Geometry: final body of the model. Coordinates: model frame, mm. Coordinates: 2 decimals unless noted, no trailing zeros. Write each loop counter-clockwise with the first axis right and the second up, starting at its lowest first coordinate (ties: lowest second). Pieces come first, ordered by that corner, then holes. Notation, with made-up numbers: (-15.75, 81) - (7.25, 81) arc R23 cw to (7.25, 104) - close; hole circle Ø5 at (70.5, 45.5). An arc over 180 degrees is marked (long way). Answer as a JSON object with one key per item and string values. Group by question number.
Item 1: Section B-B on x = -9. Return loops of the section in (y, z), and give its area (3 significant figures).
Item 2: First-contact query: pin 1 Ø2 at (x, y) = (18.5, -10.5) entering from -Z; pin 2 Ø6 at (x, y) = (12, -24) entering from +Z; pin 3 Ø8 at (x, y) = (32.5, -18.5) entering from -Z. Flat tips, straight axial feed; report the tip coordinate or a pass-through.
Item 3: Section C-C on z = -11. Return loops of the section in (x, y).
Item 4: Section A-A on y = -25.5. Return loops of the section in (x, z), and give its area (3 significant figures).
Item 5: Line query: line 1 along X through (y, z) = (-38.5, -6.5); line 2 along Z through (x, y) = (8, -37); line 3 along X through (y, z) = (-36.5, 7). Output: solid intervals per line, ascending. Write a range as from..to.
```python
from build123d import *

# Parameters (mm, degrees)
F1_DEPTH = 50.8


with BuildPart() as f1:
    # F0 (on Front) → F1 (new body)
    with BuildSketch(Plane.XZ):
        with BuildLine():
            Line((4.744167, 14.229999), (0, 15))
            ThreePointArc((0, 15), (-15, 0), (0, -15))
            Line((0, -15), (5.124627, -14.097454))
            ThreePointArc((5.124627, -14.097454), (12.285548, -8.60612), (15, 0))
            ThreePointArc((15, 0), (12.168864, 8.770333), (4.744167, 14.229999))
        make_face()
        with BuildLine():
            ThreePointArc((4.744167, 14.229999), (2.403124, 14.806248), (0, 15))
            Line((0, 15), (4.744167, 14.229999))
        make_face()
        with BuildLine():
            Line((5.124627, -14.097454), (0, -15))
            ThreePointArc((0, -15), (2.601749, -14.77264), (5.124627, -14.097454))
        make_face()
        with BuildLine():
            Line((31.602083, 9.870832), (4.744167, 14.229999))
            ThreePointArc((4.744167, 14.229999), (12.168864, 8.770333), (15, 0))
            ThreePointArc((15, 0), (12.285548, -8.60612), (5.124627, -14.097454))
            Line((5.124627, -14.097454), (28.800074, -9.927748))
            ThreePointArc((28.800074, -9.927748), (20.098668, 1.401293), (31.602083, 9.870832))
        make_face()
        with BuildLine():
            ThreePointArc((36.268126, 7.7917), (34.070104, 9.134235), (31.602083, 9.870832))
            ThreePointArc((31.602083, 9.870832), (20.098668, 1.401293), (28.800074, -9.927748))
            ThreePointArc((28.800074, -9.927748), (36.633277, -7.48329), (40, 0))
            ThreePointArc((40, 0), (39.018904, 4.319649), (36.268126, 7.7917))
        make_face()
    extrude(amount=F1_DEPTH)


solid = f1.part
```
Checks:
{
 "1": {"outline": "(-50.8, -12) - (0, -12) - (0, 12) - (-50.8, 12) - close", "area": "1,220 mm^2"},
 "2": {"pin 1": "z = -11.92", "pin 2": "z = 13.54", "pin 3": "z = -10"},
 "3": {"outline": "(-10.2, -50.8) - (22.71, -50.8) - (22.71, 0) - (-10.2, 0) - close"},
 "4": {"outline": "(0, -15) arc R15 ccw to (5.12, -14.1) - (28.8, -9.93) arc R10 ccw to (40, 0) arc R10 ccw to (36.27, 7.79) arc R10 ccw to (31.6, 9.87) - (4.74, 14.23) arc R15 ccw to (0, 15) arc R15 ccw to start", "area": "1,260 mm^2"},
 "5": {"line 1": "-13.52..37.6", "line 2": "-13.59..13.7", "line 3": "-13.27..37.14"}
}
